Check sheet for the modelled part. Datum: model origin and axes. Units: mm. A direction names the side the tool comes from. Round coordinates to 2 decimals unless told otherwise and drop trailing zeros. Write each loop counter-clockwise with the first axis right and the second up, starting at its lowest first coordinate (ties: lowest second). Pieces come first, ordered by that corner, then holes.
Item 1: Section check C-C, the plane y = -11. Record the cut outline in (x, z), plus the area to 3 significant figures.
Item 2: Section check D-D, the plane x = -6.5. Record the cut outline in (y, z), plus the area to 3 significant figures.
Item 3: Section check A-A, the plane x = 0. Record the cut outline in (y, z), plus the area to 3 significant figures.
Item 4: Release check for a two-part mould opening along X. For faces 3 (the cylindrical face through (14.985, 0.66, -1.479)), 4 (the cylindrical face through (6.03, -11.8, -1.48)), 5 (the flat face through (-3, -3, -3)) record: pulls with the +X half, pulls with the -X half, needs draft (parallel to the pull), parting line crosses it, or undercut.
Item 5: Material ranges on line 1 along Y through (x, z) = (6.25, -1.9); line 2 along Y through (x, z) = (0, -1); line 3 along Y through (x, z) = (0, 1.25), recorded low to high.
Item 6: Section check B-B, the plane y = 0. Record the cut outline in (x, z), plus the area to 3 significant figures.
Item 7: Depth check by flat-ended pin: pin 1 (4.5 mm diameter, centred on x = 0, y = 0, fed in from -Z); pin 2 (3 mm diameter, centred on x = -10, z = -1.5, fed in from +Y); pin 3 (3 mm diameter, centred on x = -12.5, y = 0, fed in from +Z); pin 4 (3 mm diameter, centred on y = -8.5, z = 0.5, fed in from -X). Enter the tip coordinate at first touch or a pass-through.
Item 8: Set-up check for faces 1 (the cylindrical face through (5.456, 10.217, -1.479)), 2 (the flat face through (0, -10, 0)): record each of +Z, -Z, +X, -X, +Y, -Y from which the full face is reachable in a straight line by a thin tool's end or side.
from build123d import *

# Parameters (mm, degrees)
SKETCH_1_R               = 9.5
EXTRUDE_1_DEPTH          = 3
SKETCH_2_R               = 15
EXTRUDE_2_DEPTH          = 3
SKETCH_3_R               = 3.9
CUT_EXTRUDE_3_DEPTH      = 23.045407685
SKETCH_4_R               = 1
CUT_EXTRUDE_4_DEPTH      = 22.424285286
PATTERN_CIRCULAR_1_COUNT = 3


with BuildPart() as part:
    # Эскиз1 → Бобышка-Вытянуть1 (new body)
    with BuildSketch(Plane.XY):
        Circle(SKETCH_1_R)
    extrude(amount=EXTRUDE_1_DEPTH)

    # Эскиз2 → Бобышка-Вытянуть2 (add)
    with BuildSketch(Plane(origin=(0, 0, 0), x_dir=(-1, 0, 0), z_dir=(0, 0, -1))):
        Circle(SKETCH_2_R)
    extrude(amount=EXTRUDE_2_DEPTH)

    # Эскиз3 → Вырез-Вытянуть3 (cut, through all)
    with BuildSketch(Plane.XY.offset(3)):
        Circle(SKETCH_3_R)
    extrude(amount=-CUT_EXTRUDE_3_DEPTH, mode=Mode.SUBTRACT)

    # Эскиз4 → Вырез-Вытянуть4 (cut, through all)
    with BuildSketch(Plane.XY):
        with Locations((-12.5, 0)):
            Circle(SKETCH_4_R)
    cut_extrude_4 = extrude(amount=-CUT_EXTRUDE_4_DEPTH, mode=Mode.SUBTRACT)

    # Круговой массив1: Вырез-Вытянуть4 ×3 about axis
    pattern_circular_1_axis = Axis((0, 0, 0), (0, 0, 1))
    for i in range(1, PATTERN_CIRCULAR_1_COUNT):
        add(cut_extrude_4.rotate(pattern_circular_1_axis, i * 360 / PATTERN_CIRCULAR_1_COUNT), mode=Mode.SUBTRACT)


solid = part.part
Values found:
1. outline: (-10.2, -3) - (5.27, -3) - (5.27, 0) - (-10.2, 0) - close; (7.23, -3) - (10.2, -3) - (10.2, 0) - (7.23, 0) - close
1. area: 55.3 mm2
2. outline: (-13.52, -3) - (13.52, -3) - (13.52, 0) - (6.93, 0) - (6.93, 3) - (-6.93, 3) - (-6.93, 0) - (-13.52, 0) - close
2. area: 123 mm2
3. outline: (-15, -3) - (-3.9, -3) - (-3.9, 3) - (-9.5, 3) - (-9.5, 0) - (-15, 0) - close; (3.9, -3) - (15, -3) - (15, 0) - (9.5, 0) - (9.5, 3) - (3.9, 3) - close
3. area: 100 mm2
4. face 3: parting line crosses it
4. face 4: undercut
4. face 5: needs draft
5. line 1: y = -13.64 to -11.83, -9.83 to 9.83, 11.83 to 13.64
5. line 2: y = -15 to -3.9, 3.9 to 15
5. line 3: y = -9.5 to -3.9, 3.9 to 9.5
6. outline: (-15, -3) - (-13.5, -3) - (-13.5, 0) - (-15, 0) - close; (-11.5, -3) - (-3.9, -3) - (-3.9, 3) - (-9.5, 3) - (-9.5, 0) - (-11.5, 0) - close; (3.9, -3) - (15, -3) - (15, 0) - (9.5, 0) - (9.5, 3) - (3.9, 3) - close
6. area: 94.2 mm2
7. pin 1: passes through
7. pin 2: stops at y = 12.36
7. pin 3: stops at z = 0
7. pin 4: stops at x = -13.22
8. face 1: +Z, -Z
8. face 2: +Z
